Autodesk Inventor part; units mm, degrees
ref_plane "YZ Plane" through (0, 0, 0) normal (1, 0, 0) x (0, 1, 0)
ref_plane "XZ Plane" through (0, 0, 0) normal (0, 1, 0) x (-1, 0, 0)
ref_plane "XY Plane" through (0, 0, 0) normal (0, 0, 1) x (1, 0, 0)
sketch "Sketch1" plane through (0, 0, 0) normal (0, 0, 1) x (1, 0, 0)
  line L0 (-106.045, 6.985) -> (-90.7112, 6.985)
  line L1 (-88.1712, 6.985) -> (-72.8375, 6.985)
  line L2 (-72.8375, 6.985) -> (-72.8375, 19.492)
  line L3 (-106.045, 19.492) -> (-106.045, 6.985)
  line L4 (-106.045, 19.492) -> (-72.8375, 19.492)
  line L5 (-90.0762, 5.207) -> (-88.8062, 5.207)
  line L6 (-88.1712, 6.985) -> (-88.1712, 5.842)
  line L7 (-90.7112, 6.985) -> (-90.7112, 5.842)
  arc A0 (-90.7112, 5.842) -> (-90.0762, 5.207) centre (-90.0762, 5.842) ccw
  arc A1 (-88.8062, 5.207) -> (-88.1712, 5.842) centre (-88.8062, 5.842) ccw
  point P0 (0, 0)
  dimension "d0" = 0.635
extrude "Extrusion1" add sketch "Sketch1" along normal blind 1.27
fillet "Fillet1" radius 0.635 10 edges at (-88.3572, 5.393, 0) (-89.4412, 5.207, 0) (-90.5253, 5.393, 0) (-90.7112, 6.4135, 0) (-88.1712, 6.4135, 0) (-88.3572, 5.393, 1.27) (-89.4412, 5.207, 1.27) (-90.5253, 5.393, 1.27) (-90.7112, 6.4135, 1.27) (-88.1712, 6.4135, 1.27)
sketch "Sketch2" plane through (0, 0, 1.27) normal (0, 0, 1) x (1, 0, 0)
  line L0 (-72.8375, 19.492) -> (-106.045, 19.492)
  line L1 (-72.8375, 19.492) -> (-106.045, 19.492)
  line L2 (-89.4412, 19.492) -> (-89.4412, 18.222)
  line L3 (-89.4412, 18.222) -> (-91.3462, 18.222)
  line L4 (-91.3462, 18.222) -> (-91.3462, 19.492)
  line L5 (-89.4412, 18.222) -> (-87.5362, 18.222)
  line L6 (-87.5362, 18.222) -> (-87.5362, 19.492)
  line L7 (-91.3462, 19.492) -> (-87.5362, 19.492)
  point P0 (0, 0)
  dimension "d4" = 1.27
  dimension "d5" = 1.905
  dimension "d6" = 1.905
extrude "Extrusion2" add sketch "Sketch2" along normal blind 3.81
fillet "Fillet2" radius 0.635 4 edges at (-89.4412, 19.492, 5.08) (-89.4412, 18.222, 5.08) (-87.5362, 18.857, 1.27) (-91.3462, 18.857, 1.27)
properties part number "FloppyCover" material "UHMW, Black"
Verification items for the finished model (mm, model axes). A direction names the side the tool comes from. Round coordinates to 2 decimals unless told otherwise and drop trailing zeros. Write each loop counter-clockwise with the first axis right and the second up, starting at its lowest first coordinate (ties: lowest second). Pieces come first, ordered by that corner, then holes.
1. Gauge pin test, flat ends, axial feed: P1, Ø1.4, axis at y = 19, z = 4, coming from the -X side; P2, Ø8, axis at x = -80, y = 16.5, coming from the -Z side; P3, Ø1, axis at y = 19, z = 3.5, coming from the +X side; P4, Ø1.4, axis at x = -83.5, z = 1, coming from the -Y side (3 decimals). Record the tip position at first contact, or that the pin passes through.
2. Section check A-A on x = -81. Enter the section's corners in (y, z) (3 decimals), plus the area to 3 significant figures.
3. Scan lines: L1, parallel to Z at x = -104, y = 18.5; L2, parallel to Y at x = -88.5, z = 4.45; L3, parallel to Y at x = -90.5, z = 4.8. Record each from-to range of solid material in increasing order.
4. Section check B-B on y = 16.5. Enter the section's corners in (x, z) (1 decimal).
5. Access from +Z, -Z, +X, -X, +Y, -Y to the whole of each face (thin tool, end or side, straight path). Record for faces 1 (the flat face through (-106.045, 13, 1)), 2 (the flat face through (-91.346, 19, 3)), 3 (the flat face through (-90, 19.492, 1)), 4 (the flat face through (-89, 18.222, 3)), 5 (the flat face through (-87.536, 19, 3)).
Answer:
1. P1: stops at x = -91.35
1. P2: stops at z = 0
1. P3: stops at x = -87.54
1. P4: stops at y = 6.985
2. outline: (6.985, 0) - (19.492, 0) - (19.492, 1.27) - (6.985, 1.27) - close
2. area: 15.9 mm2
3. L1: z = 0 to 1.27
3. L2: y = 18.22 to 19.49
3. L3: y = 18.33 to 19.38
4. outline: (-106, 0) - (-72.8, 0) - (-72.8, 1.3) - (-106, 1.3) - close
5. face 1: +Z, -Z, -X, +Y, -Y
5. face 2: +Z, -X, +Y, -Y
5. face 3: +Z, -Z, +X, -X, +Y
5. face 4: +Z, +X, -X, -Y
5. face 5: +Z, +X, +Y, -Y
